Geometry: final body of the model. Coordinates: model frame, mm. Face numbers are marked on the shaded views. A direction names the side the tool comes from. Give positions to 0.01 mm unless a question says otherwise; leave off trailing zeros. Write each loop counter-clockwise with the first axis right and the second up, starting at its lowest first coordinate (ties: lowest second). Pieces come first, ordered by that corner, then holes. Notation, with made-up numbers: (36.25, 13.5) - (81.25, 13.5) arc R27 ccw to (81.25, 31.5) - close; hole circle Ø7 at (26, -10). An arc over 180 degrees is marked (long way). Use CSV: the item, a comma, the result in double quotes. Start each with the question number.
(1) Section C-C on z = 3. Output: boundary loops of the cut face in (x, y), and give its area (3 significant figures).
(2) Line query: probe 1 along Z at (x, y) = (1.2, 1.75); probe 2 along X at (y, z) = (-0.1, 5); probe 3 along Y at (x, z) = (0.15, 0.5). Output: solid intervals per line, ascending. Write a range as [from, to].
(3) Reachability of the marked faces 1, 2 and 3 from +Z, -Z, +X, -X, +Y, -Y: full face, straight path, thin tool, end or side. Return the list, or none.
(4) First-contact query: pin 1 Ø1 at (y, z) = (1.5, -21) entering from +X. Flat tip, straight axial feed; report the tip coordinate or a pass-through.
(5) Section A-A on x = 0. Output: boundary loops of the cut face in (y, z).
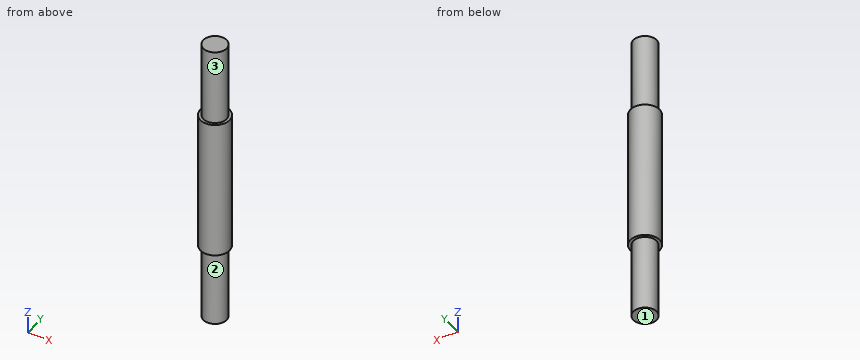
from build123d import *

# Parameters (mm, degrees)
ESQUISSE1_R        = 2.5
BOSS_EXTRU_1_DEPTH = 24
ESQUISSE2_R        = 2
BOSS_EXTRU_2_DEPTH = 13
BOSS_EXTRU_3_START = 13
ESQUISSE3_R        = 2
BOSS_EXTRU_3_DEPTH = 13


with BuildPart() as part:
    # Esquisse1 → Boss.-Extru.1 (new body)
    with BuildSketch(Plane.XY):
        Circle(ESQUISSE1_R)
    extrude(amount=-BOSS_EXTRU_1_DEPTH)

    # Esquisse2 → Boss.-Extru.2 (add)
    with BuildSketch(Plane.XY):
        with Locations(Location((0, 0, 0), (0, 0, 180))):
            Circle(ESQUISSE2_R)
    extrude(amount=BOSS_EXTRU_2_DEPTH)

    # Esquisse3 → Boss.-Extru.3 (add)
    with BuildSketch(Plane(origin=(0, 0, -24), x_dir=(-1, 0, 0), z_dir=(0, 0, -1)).offset(BOSS_EXTRU_3_START)):
        Circle(ESQUISSE3_R)
    extrude(amount=-BOSS_EXTRU_3_DEPTH)


solid = part.part
Check values:
1,outline,"circle Ø4 at (0, 0)"
1,area,"12.6 mm²"
2,probe 1,"z = [-24, 0]"
2,probe 2,"x = [-2, 2]"
2,probe 3,"y = [-1.99, 1.99]"
3,face 1,"-Z, +X, -X, +Y, -Y"
3,face 2,"-Z"
3,face 3,"+Z"
4,pin 1,"stops at x = 2.29"
5,outline,"(-2.5, -24) - (-2, -24) - (-2, -37) - (2, -37) - (2, -24) - (2.5, -24) - (2.5, 0) - (2, 0) - (2, 13) - (-2, 13) - (-2, 0) - (-2.5, 0) - close"
